Geometry: see drawing. Coordinates: mm, zero at the bounding-box minimum. A direction names the side the tool comes from. Round coordinates to 2 decimals unless told otherwise and drop trailing zeros. Loops run counter-clockwise (first coordinate to the right, second up) from the corner with the lowest first, then second, coordinate; pieces in that order, holes last. Notation, with made-up numbers: (20.5, 48.25) - (27.5, 48.25) arc R22 cw to (27.5, 57.25) - close; hole circle Ø4 at (84, 6.25). An arc over 180 degrees is marked (long way). Answer in a Markdown table with one row per item. Add a question column.
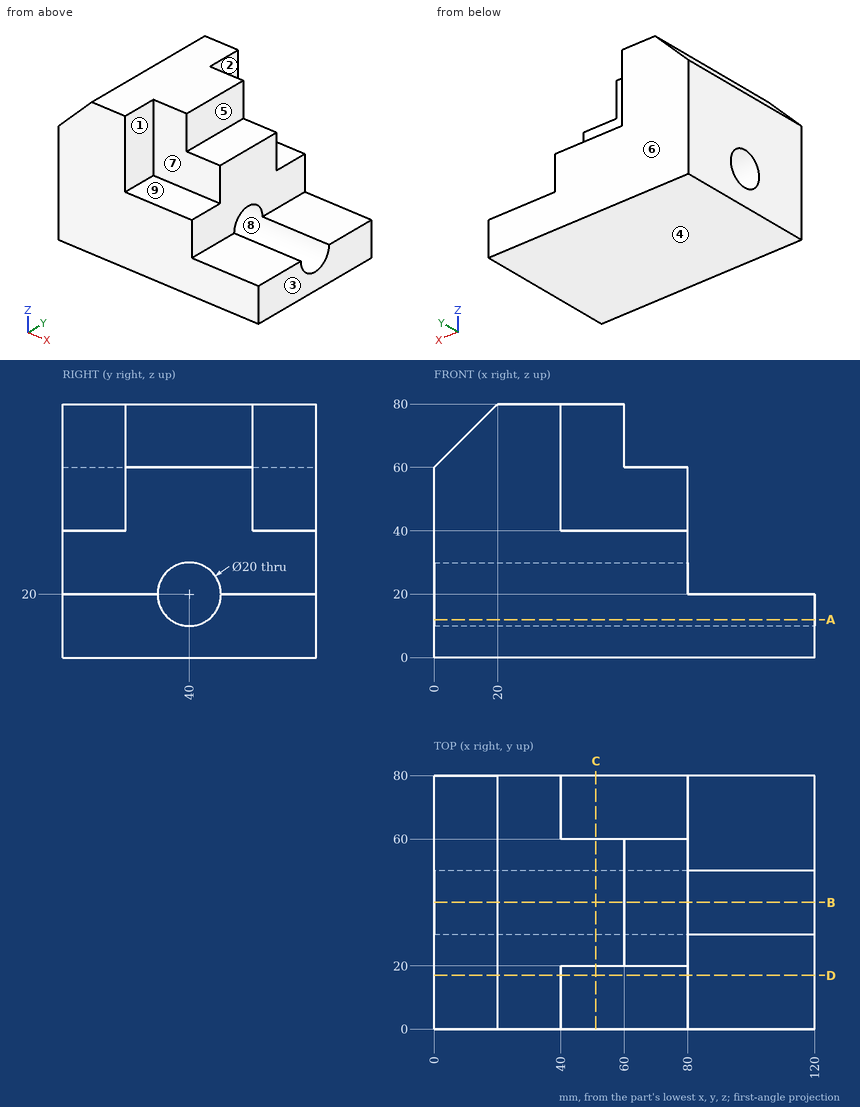
1) Section D-D, the plane y = 17. Return the cut outline in (x, z).
2) Section B-B, the plane y = 40. Return the cut outline in (x, z).
3) Reachability of the marked faces 1, 2, 3, 4 and 5 from +Z, -Z, +X, -X, +Y, -Y: full face, straight path, thin tool, end or side. Return the list, or none.
4) Section A-A, the plane z = 12. Return the cut outline in (x, y), and give its area (3 significant figures).
5) Pull-direction query (Y, two-part tool) for the marked faces 6, 7, 8 and 9; classes: pulls with the +Y half, pulls with the -Y half, needs draft (parallel to the pull), parting line crosses it, or undercut.
6) Section C-C, the plane x = 51. Return the cut outline in (y, z), and give its area (3 significant figures).
7) Contact query for flat-ended pins moving along their axis: pin 1 Ø4 at (x, z) = (65, 11.5) entering from -Y; pin 2 Ø16 at (x, y) = (71, 43) entering from +Z; pin 3 Ø15 at (x, y) = (93.5, 62.5) entering from +Z; pin 4 Ø20 at (y, z) = (60, 41.5) entering from +X. Output: stop coordinate, or through.
8) Material intervals for line 1 along Z through (x, y) = (45, 40); line 2 along Y through (x, z) = (34, 20); line 3 along X through (y, z) = (22.5, 58.5), sorted ascending. Write a range as from..to.
Evaluation:
| question | item | result |
|---|---|---|
| 1 | outline | (0, 0) - (120, 0) - (120, 20) - (80, 20) - (80, 40) - (40, 40) - (40, 80) - (20, 80) - (0, 60) - close |
| 2 | outline | (0, 0) - (120, 0) - (120, 10) - (0, 10) - close; (0, 30) - (80, 30) - (80, 60) - (60, 60) - (60, 80) - (20, 80) - (0, 60) - close |
| 3 | face 1 | +Z, +X, -Y |
| 3 | face 2 | +Z, +X, +Y |
| 3 | face 3 | +Z, -Z, +X, +Y, -Y |
| 3 | face 4 | -Z, +X, -X, +Y, -Y |
| 3 | face 5 | +Z, +X, +Y, -Y |
| 4 | outline | (0, 0) - (120, 0) - (120, 34) - (0, 34) - close; (0, 46) - (120, 46) - (120, 80) - (0, 80) - close |
| 4 | area | 8,160 mm² |
| 5 | face 6 | pulls with the +Y half |
| 5 | face 7 | pulls with the -Y half |
| 5 | face 8 | undercut |
| 5 | face 9 | needs draft |
| 6 | outline | (0, 0) - (80, 0) - (80, 40) - (60, 40) - (60, 80) - (20, 80) - (20, 40) - (0, 40) - close; hole circle Ø20 at (40, 20) |
| 6 | area | 4,490 mm² |
| 7 | pin 1 | stops at y = 0 |
| 7 | pin 2 | stops at z = 60 |
| 7 | pin 3 | stops at z = 20 |
| 7 | pin 4 | stops at x = 80 |
| 8 | line 1 | z = 0..10, 30..80 |
| 8 | line 2 | y = 0..30, 50..80 |
| 8 | line 3 | x = 0..80 |
